from build123d import *

# Parameters (mm, degrees)
SALIENTE_EXTRUIR1_DEPTH = 10
CROQUIS2_R              = 5
CORTAR_EXTRUIR1_DEPTH   = 10


with BuildPart() as part:
    # Croquis1 → Saliente-Extruir1 (new body)
    with BuildSketch(Plane(origin=(0, 0, 0), x_dir=(1, 0, 0), z_dir=(0, 1, 0))):
        with BuildLine():
            Line((-25, -25), (25, -25))
            Line((25, -25), (25, -24.43130904))
            ThreePointArc((25, -24.43130904), (10.521904785, 10.521904785), (-24.43130904, 25))
            Line((-24.43130904, 25), (-25, 25))
            Line((-25, 25), (-25, -25))
        make_face()
    extrude(amount=SALIENTE_EXTRUIR1_DEPTH)

    # Croquis2 → Cortar-Extruir1 (cut)
    with BuildSketch(Plane(origin=(0, 10, 0), x_dir=(1, 0, 0), z_dir=(0, 1, 0))):
        with Locations(Location((0, 0, 0), (0, 0, 270))):
            Circle(CROQUIS2_R)
    extrude(amount=-CORTAR_EXTRUIR1_DEPTH, mode=Mode.SUBTRACT)


solid = part.part
Could you check a few things on this model? Use its own coordinates, in mm. Give positions to 0.01 mm unless a question says otherwise; leave off trailing zeros. Order: outer loops, then holes, each group sorted by start corner. A loop starts at its lowest first (then second) coordinate and runs counter-clockwise, first axis right, second up. Notation, with made-up numbers: (13, -32.75) -> (70, -32.75) arc R29 ccw to (70, 0.25) -> close; hole circle Ø11 at (-6, 86.5). An arc over 180 degrees is marked (long way). Answer in a Markdown table with one row per item. Add a question column.
Item 1: Imagine slicing it at C-C (x = 0). List the corners of the cut face in (y, z) for me, and give its area (3 significant figures).
Item 2: Imagine slicing it at B-B (z = 0). List the corners of the cut face in (x, y) for me, and give its area (3 significant figures).
Item 3: We'd pull the mould along Z, two halves only. Please class faces 1 (the flat face through (0, 5, 25)), 2 (the flat face through (-6, 0, 5)), 3 (the cylindrical face through (-4.88, 5.07, -1.08)): pulls with the +Z half, pulls with the -Z half, needs draft (parallel to the pull), parting line crosses it, or undercut.
Item 4: I'm going to push flat-ended pins straight in: P1, Ø13, axis at x = 0, z = 0, coming from the -Y side; P2, Ø2, axis at x = 12.5, y = 2.5, coming from the -Z side; P3, Ø4, axis at x = -14, y = 8, coming from the -Z side; P4, Ø5, axis at x = 0.5, y = 6.5, coming from the -Z side. Where does each tip first touch, or does it pass through?
Item 5: Imagine slicing it at D-D (x = 7.5). List the corners of the cut face in (y, z) for me, and give its area (3 significant figures).
Item 6: Imagine slicing it at A-A (y = 6.25). List the corners of the cut face in (x, z) for me.
Item 7: Please list where these lines run through material, in increasing order: probe 1 along X at (y, z) = (6.5, 0); probe 2 along X at (y, z) = (7.5, -1.5); probe 3 along Z at (x, y) = (4.5, 2.5).
Result:
| question | item | result |
|---|---|---|
| 1 | outline | (0, -18.54) -> (10, -18.54) -> (10, -5) -> (0, -5) -> close; (0, 5) -> (10, 5) -> (10, 25) -> (0, 25) -> close |
| 1 | area | 335 mm2 |
| 2 | outline | (-25, 0) -> (-5, 0) -> (-5, 10) -> (-25, 10) -> close; (5, 0) -> (18.54, 0) -> (18.54, 10) -> (5, 10) -> close |
| 2 | area | 335 mm2 |
| 3 | face 1 | pulls with the +Z half |
| 3 | face 2 | needs draft |
| 3 | face 3 | undercut |
| 4 | P1 | y = 0 |
| 4 | P2 | z = -9.52 |
| 4 | P3 | z = -24.28 |
| 4 | P4 | z = -19.62 |
| 5 | outline | (0, -13.3) -> (10, -13.3) -> (10, 25) -> (0, 25) -> close |
| 5 | area | 383 mm2 |
| 6 | outline | (-25, -25) -> (-24.43, -25) arc R49.43 ccw to (25, 24.43) -> (25, 25) -> (-25, 25) -> close; hole circle Ø10 at (0, 0) |
| 7 | probe 1 | -25 to -5, 5 to 18.54 |
| 7 | probe 2 | -25 to -4.77, 4.77 to 17.65 |
| 7 | probe 3 | -15.65 to -2.18, 2.18 to 25 |
